Verification items for the finished model (mm, model axes). A direction names the side the tool comes from. Coordinates: 2 decimals unless noted, no trailing zeros. Write each loop counter-clockwise with the first axis right and the second up, starting at its lowest first coordinate (ties: lowest second). Pieces come first, ordered by that corner, then holes. Notation, with made-up numbers: (11, 88) -> (55, 88) arc R25 cw to (55, 125) -> close; hole circle Ø8 at (58.25, 26.25). An arc over 180 degrees is marked (long way). Write item = value, one per line. Start each with the question number.
(1) Material ranges on probe 1 along Z at (x, y) = (-40, 76); probe 2 along Z at (x, y) = (-40, 78.5); probe 3 along X at (y, z) = (81, -30), recorded low to high. Write a range as [from, to].
(2) Set-up check for faces 1 (the face through (55.21, 66.115, 112.168)), 2 (the face through (70, 76, 110)), 3 (the face through (-29.58, 66.956, -34.614)): record each of +Z, -Z, +X, -X, +Y, -Y from which the full face is reachable in a straight line by a thin tool's end or side.
(3) Mould release check, pull along Z, two halves, no side actions. Record for faces 4 (the face through (20, 76, -60)), 5 (the face through (-60, 76, -30)), 6 (the face through (-34.51, 72.05, 100.76)): released by +Z, released by -Z, zero draft, split by the parting line, or undercut.
(4) Section check A-A (z = -30). Record the cut outline in (x, y).
(5) Section check B-B (x = -40). Record the cut outline in (y, z), plus the area to 3 significant figures.
(6) Section check D-D (z = 110). Record the cut outline in (x, y).
(7) Gauge pin test, flat ends, axial feed: pin 1 Ø6 at (x, y) = (-14.5, 61.5) entering from +Z; pin 2 Ø5 at (x, y) = (-51, 82) entering from -Z; pin 3 Ø2 at (x, y) = (-22, 78.5) entering from +Z; pin 4 Ø6 at (y, z) = (74, -34.5) entering from -X. Record the tip position at first contact, or that the pin passes through.
(8) Section check C-C (y = 80.5). Record the cut outline in (x, z).
```python
from build123d import *

# Parameters (mm, degrees)
SKETCH1_W           = 210
SKETCH1_H           = 38.1
BOSS_EXTRUDE1_DEPTH = 40
BOSS_EXTRUDE2_START = 30
SKETCH4_R           = 10
BOSS_EXTRUDE2_DEPTH = 140
CUT_EXTRUDE2_REACH  = 96.928
SKETCH5_R           = 4
BOSS_EXTRUDE3_START = 30
SKETCH2_R           = 10
BOSS_EXTRUDE3_DEPTH = 130
CUT_EXTRUDE3_REACH  = 96.928
SKETCH6_R           = 4


with BuildPart() as part:
    # Sketch1 → Boss-Extrude1 (new body)
    with BuildSketch(Plane(origin=(0, 0, 0), x_dir=(0, 0, -1), z_dir=(1, 0, 0))):
        with Locations((-45, 75.877536232)):
            Rectangle(SKETCH1_W, SKETCH1_H)
    extrude(amount=BOSS_EXTRUDE1_DEPTH)

    # Sketch4 → Boss-Extrude2 (add)
    with BuildSketch(Plane(origin=(40, 0, 0), x_dir=(0, 0, -1), z_dir=(1, 0, 0)).offset(BOSS_EXTRUDE2_START)):
        with Locations((-110, 75.877536232)):
            Circle(SKETCH4_R)
    extrude(amount=-BOSS_EXTRUDE2_DEPTH)

    # Sketch5 → Cut-Extrude2 (cut, up to next)
    with BuildSketch(Plane(origin=(0, 0, 0), x_dir=(1, 0, 0), z_dir=(0, 1, 0)), mode=Mode.PRIVATE) as cut_extrude2_sk1:
        with Locations((-60, -110)):
            Circle(SKETCH5_R)
    cut_extrude2_tool1 = extrude(cut_extrude2_sk1.sketch, amount=CUT_EXTRUDE2_REACH, mode=Mode.PRIVATE) & part.part
    add(cut_extrude2_tool1.solids().sort_by_distance((-60, 0, 110))[0], mode=Mode.SUBTRACT)

    # Sketch2 → Boss-Extrude3 (add)
    with BuildSketch(Plane(origin=(40, 0, 0), x_dir=(0, 0, -1), z_dir=(1, 0, 0)).offset(BOSS_EXTRUDE3_START)):
        with Locations((30, 75.827536232)):
            Circle(SKETCH2_R)
    extrude(amount=-BOSS_EXTRUDE3_DEPTH)

    # Sketch6 → Cut-Extrude3 (cut, up to next)
    with BuildSketch(Plane(origin=(0, 0, 0), x_dir=(1, 0, 0), z_dir=(0, 1, 0)), mode=Mode.PRIVATE) as cut_extrude3_sk1:
        with Locations((-40, 30)):
            Circle(SKETCH6_R)
    cut_extrude3_tool1 = extrude(cut_extrude3_sk1.sketch, amount=CUT_EXTRUDE3_REACH, mode=Mode.PRIVATE) & part.part
    add(cut_extrude3_tool1.solids().sort_by_distance((-40, 0, -30))[0], mode=Mode.SUBTRACT)


solid = part.part
```
Response:
q1.probe_1 = [-40, -34], [-26, -20], [100, 120]
q1.probe_2 = [-39.64, -34], [-26, -20.36], [100.35, 119.65]
q1.probe_3 = [-60, -44], [-36, 70]
q2.face_1 = +X
q2.face_2 = +Z, -Z, +X, +Y, -Y
q2.face_3 = -X
q3.face_4 = released by -Z
q3.face_5 = zero draft
q3.face_6 = undercut
q4.outline = (-60, 65.83) -> (-44, 65.83) -> (-44, 85.83) -> (-60, 85.83) -> close; (-36, 65.83) -> (0, 65.83) -> (0, 56.83) -> (40, 56.83) -> (40, 65.83) -> (70, 65.83) -> (70, 85.83) -> (40, 85.83) -> (40, 94.93) -> (0, 94.93) -> (0, 85.83) -> (-36, 85.83) -> close
q5.outline = circle Ø20 at (75.88, 110); (66.66, -34) arc R10 ccw to (84.99, -34) -> close; (66.66, -26) -> (84.99, -26) arc R10 ccw to start
q5.area = 473 mm2
q6.outline = (-70, 65.88) -> (-64, 65.88) -> (-64, 85.88) -> (-70, 85.88) -> close; (-56, 65.88) -> (0, 65.88) -> (0, 56.83) -> (40, 56.83) -> (40, 65.88) -> (70, 65.88) -> (70, 85.88) -> (40, 85.88) -> (40, 94.93) -> (0, 94.93) -> (0, 85.88) -> (-56, 85.88) -> close
q7.pin_1 = through
q7.pin_2 = -39.3
q7.pin_3 = 119.87
q7.pin_4 = -60
q8.outline = (-70, 101.13) -> (0, 101.13) -> (0, -21.16) -> (-60, -21.16) -> (-60, -38.84) -> (0, -38.84) -> (0, -60) -> (40, -60) -> (40, -38.84) -> (70, -38.84) -> (70, -21.16) -> (40, -21.16) -> (40, 101.13) -> (70, 101.13) -> (70, 118.87) -> (40, 118.87) -> (40, 150) -> (0, 150) -> (0, 118.87) -> (-70, 118.87) -> close; hole circle Ø8 at (-60, 110); hole circle Ø8 at (-40, -30)
